Build history of the part. All positions in model axes, mm. A direction names the side the tool comes from. Round coordinates to 2 decimals unless told otherwise and drop trailing zeros. Order: outer loops, then holes, each group sorted by start corner. A loop starts at its lowest first (then second) coordinate and runs counter-clockwise, first axis right, second up. Notation, with made-up numbers: (-38.75, -3) -> (-14.75, -3) arc R18 cw to (-14.75, 11) -> close; hole circle Ø5 at (42.5, 11). An arc over 180 degrees is marked (long way). Use a Markdown table: item, result. Add a question column.
Item 1: Probe L1, parallel to X at y = 13.5, z = -88; L2, parallel to Z at x = 91, y = 7; L3, parallel to X at y = 25, z = -105. List the from-to ranges inside material, lowest first.
Item 2: Two-plate mould, pull along X, no slides. Class faces 6 (the face through (1, 4, -74)), 7 (the face through (74, 35, -54)): released by +X, released by -X, zero draft, split by the parting line, or undercut.
Item 3: Slice it at B-B, the plane z = -33. Give the cut face in (x, y).
Item 4: Pin check, flat tips, straight feed: pin 1 (2.5 mm diameter, centred on x = 1, y = 4.5, fed in from +Z); pin 2 (2 mm diameter, centred on y = 11, z = -59.5, fed in from -X); pin 3 (16 mm diameter, centred on x = 12, y = 8.5, fed in from +Z); pin 4 (1.2 mm diameter, centred on x = 29.5, z = -104.5, fed in from -Y). Stop position of each tip, or through.
Item 5: Slice it at A-A, the plane x = 62.5. Give the cut face in (y, z), plus the area to 3 significant figures.
Item 6: Slice it at D-D, the plane z = -53. Give the cut face in (x, y), plus the area to 3 significant figures.
Item 7: 3-axis set-ups, long thin cutter, end or side, ignore diameter. For faces 1 (the face through (5, 16, -106)), 2 (the face through (125, 16, -9)), 3 (the face through (1.52, 21.88, -86.65)), 4 (the face through (125, 35, -5)), 5 (the face through (59, 20.62, -1)): which of +Z, -Z, +X, -X, +Y, -Y reach the whole face in a straight line?
Item 8: Slice it at C-C, the plane x = 102.5. Give the cut face in (y, z), plus the area to 3 significant figures.
from build123d import *

# Parameters (mm, degrees)
SKETCH1_W           = 150
SKETCH1_H           = 110
BOSS_EXTRUDE1_DEPTH = 38
SKETCH3_W           = 144
SKETCH3_H           = 104
CUT_EXTRUDE1_DEPTH  = 35
CUT_EXTRUDE2_REACH  = 191.853
SKETCH5_W           = 10.5
SKETCH5_H           = 8.5
FILLET4_R           = 3
CUT_EXTRUDE3_REACH  = 191.853
SKETCH6_W           = 34.1
SKETCH6_H           = 45.2
CUT_EXTRUDE4_REACH  = 191.853
SKETCH10_W          = 15.12
SKETCH10_H          = 13.75
FILLET5_R           = 2
BOSS_EXTRUDE2_REACH = 191.853
SKETCH12_W          = 9
SKETCH12_H          = 6
SKETCH13_R          = 2.032
CUT_EXTRUDE5_DEPTH  = 35
CUT_EXTRUDE6_REACH  = 191.853
SKETCH14_W          = 28.8
SKETCH14_H          = 11
FILLET6_R           = 5
FILLET7_R           = 2
FILLET8_DEPTH       = 35
FILLET8_2_DEPTH     = 36
FILLET9_R           = 3


with BuildPart() as part:
    # Sketch1 → Boss-Extrude1 (new body)
    with BuildSketch(Plane(origin=(0, 0, 0), x_dir=(1, 0, 0), z_dir=(0, 1, 0))):
        with Locations((75, 55)):
            Rectangle(SKETCH1_W, SKETCH1_H)
    extrude(amount=BOSS_EXTRUDE1_DEPTH)

    # Sketch3 → Cut-Extrude1 (cut)
    with BuildSketch(Plane.XZ):
        with Locations((75, -55)):
            Rectangle(SKETCH3_W, SKETCH3_H)
    extrude(amount=-CUT_EXTRUDE1_DEPTH, mode=Mode.SUBTRACT)

    # Sketch5 → Cut-Extrude2 (cut, up to next)
    with BuildSketch(Plane.ZY, mode=Mode.PRIVATE) as cut_extrude2_sk1:
        with Locations((-91, 25.27)):
            Rectangle(SKETCH5_W, SKETCH5_H)
    cut_extrude2_tool1 = extrude(cut_extrude2_sk1.sketch, amount=-CUT_EXTRUDE2_REACH, mode=Mode.PRIVATE) & part.part
    add(cut_extrude2_tool1.solids().sort_by_distance((0, 25.27, -91))[0], mode=Mode.SUBTRACT)

    # Fillet4
    fillet4_edges = [part.edges().sort_by_distance(p)[0] for p in [
        (1.5, 21.02, -85.75),
        (1.5, 29.52, -85.75),
        (1.5, 29.52, -96.25),
        (1.5, 21.02, -96.25),
    ]]
    fillet(fillet4_edges, radius=FILLET4_R)

    # Sketch6 → Cut-Extrude3 (cut, up to next)
    with BuildSketch(Plane(origin=(0, 38, 0), x_dir=(1, 0, 0), z_dir=(0, 1, 0)), mode=Mode.PRIVATE) as cut_extrude3_sk1:
        with Locations((17.05, 22.6)):
            Rectangle(SKETCH6_W, SKETCH6_H)
    cut_extrude3_tool1 = extrude(cut_extrude3_sk1.sketch, amount=-CUT_EXTRUDE3_REACH, mode=Mode.PRIVATE) & part.part
    add(cut_extrude3_tool1.solids().sort_by_distance((17.05, 38, -22.6))[0], mode=Mode.SUBTRACT)

    # Sketch10 → Cut-Extrude4 (cut, up to next)
    with BuildSketch(Plane.XY, mode=Mode.PRIVATE) as cut_extrude4_sk1:
        with Locations((59.48, 13.745)):
            Rectangle(SKETCH10_W, SKETCH10_H)
    cut_extrude4_tool1 = extrude(cut_extrude4_sk1.sketch, amount=-CUT_EXTRUDE4_REACH, mode=Mode.PRIVATE) & part.part
    add(cut_extrude4_tool1.solids().sort_by_distance((59.48, 13.745, 0))[0], mode=Mode.SUBTRACT)

    # Fillet5
    fillet5_edges = [part.edges().sort_by_distance(p)[0] for p in [
        (51.92, 6.87, -1.5),
        (51.92, 20.62, -1.5),
        (67.04, 20.62, -1.5),
        (67.04, 6.87, -1.5),
    ]]
    fillet(fillet5_edges, radius=FILLET5_R)

    # Sketch12 → Boss-Extrude2 (add, up to next)
    with BuildSketch(Plane.XZ, mode=Mode.PRIVATE) as boss_extrude2_sk1:
        with Locations((125, -6)):
            Rectangle(SKETCH12_W, SKETCH12_H)
    boss_extrude2_tool1 = extrude(boss_extrude2_sk1.sketch, amount=-BOSS_EXTRUDE2_REACH, mode=Mode.PRIVATE) - part.part
    # Sketch12 → Boss-Extrude2 (add, up to next)
    with BuildSketch(Plane.XZ, mode=Mode.PRIVATE) as boss_extrude2_sk2:
        with Locations((30, -104)):
            Rectangle(SKETCH12_W, SKETCH12_H)
    boss_extrude2_tool2 = extrude(boss_extrude2_sk2.sketch, amount=-BOSS_EXTRUDE2_REACH, mode=Mode.PRIVATE) - part.part
    # Sketch12 → Boss-Extrude2 (add, up to next)
    with BuildSketch(Plane.XZ, mode=Mode.PRIVATE) as boss_extrude2_sk3:
        with Locations((125, -104)):
            Rectangle(SKETCH12_W, SKETCH12_H)
    boss_extrude2_tool3 = extrude(boss_extrude2_sk3.sketch, amount=-BOSS_EXTRUDE2_REACH, mode=Mode.PRIVATE) - part.part
    add(boss_extrude2_tool1.solids().sort_by_distance((125, 0, -6))[0])
    add(boss_extrude2_tool2.solids().sort_by_distance((30, 0, -104))[0])
    add(boss_extrude2_tool3.solids().sort_by_distance((125, 0, -104))[0])

    # Sketch13 → Cut-Extrude5 (cut)
    with BuildSketch(Plane.XZ):
        with Locations(Location((125, -5, 0), (0, 0, 270))):
            Circle(SKETCH13_R)
        with Locations(Location((125, -105, 0), (0, 0, 270))):
            Circle(SKETCH13_R)
        with Locations(Location((30, -105, 0), (0, 0, 270))):
            Circle(SKETCH13_R)
    extrude(amount=-CUT_EXTRUDE5_DEPTH, mode=Mode.SUBTRACT)

    # Sketch14 → Cut-Extrude6 (cut, up to next)
    with BuildSketch(Plane.ZY, mode=Mode.PRIVATE) as cut_extrude6_sk1:
        with Locations((-59.6, 5.5)):
            Rectangle(SKETCH14_W, SKETCH14_H)
    cut_extrude6_tool1 = extrude(cut_extrude6_sk1.sketch, amount=-CUT_EXTRUDE6_REACH, mode=Mode.PRIVATE) & part.part
    add(cut_extrude6_tool1.solids().sort_by_distance((0, 5.5, -59.6))[0], mode=Mode.SUBTRACT)

    # Fillet6
    fillet6_edges = [part.edges().sort_by_distance(p)[0] for p in [
        (147, 17.5, -3),
        (147, 17.5, -107),
        (3, 17.5, -107),
        (34.1, 36.5, -45.2),
        (0, 19, -110),
        (150, 19, -110),
        (150, 19, 0),
    ]]
    fillet(fillet6_edges, radius=FILLET6_R)

    # Fillet7
    fillet7_edges = [part.edges().sort_by_distance(p)[0] for p in [
        (1.5, 11, -74),
        (1.5, 11, -45.2),
    ]]
    fillet(fillet7_edges, radius=FILLET7_R)

    # Fillet8: read off the stored shape, not the designer's step
    # Fillet8 outline → Fillet8 (cut)
    with BuildSketch(Plane(origin=(0, 0, 0), x_dir=(1, 0, 0), z_dir=(0, 1, 0))):
        with BuildLine():
            Line((129.5, 101), (129.5, 104))
            ThreePointArc((129.5, 104), (128.621320344, 101.878679656), (126.5, 101))
            Line((126.5, 101), (129.5, 101))
        make_face()
        with BuildLine():
            Line((25.5, 101), (28.5, 101))
            ThreePointArc((28.5, 101), (26.378679656, 101.878679656), (25.5, 104))
            Line((25.5, 104), (25.5, 101))
        make_face()
        with BuildLine():
            Line((34.5, 101), (34.5, 104))
            ThreePointArc((34.5, 104), (33.621320344, 101.878679656), (31.5, 101))
            Line((31.5, 101), (34.5, 101))
        make_face()
        with BuildLine():
            Line((120.5, 101), (123.5, 101))
            ThreePointArc((123.5, 101), (121.378679656, 101.878679656), (120.5, 104))
            Line((120.5, 104), (120.5, 101))
        make_face()
        with BuildLine():
            Line((120.5, 9), (120.5, 6))
            ThreePointArc((120.5, 6), (121.378679656, 8.121320344), (123.5, 9))
            Line((123.5, 9), (120.5, 9))
        make_face()
        with BuildLine():
            Line((129.5, 9), (126.5, 9))
            ThreePointArc((126.5, 9), (128.621320344, 8.121320344), (129.5, 6))
            Line((129.5, 6), (129.5, 9))
        make_face()
    extrude(amount=FILLET8_DEPTH, mode=Mode.SUBTRACT)

    # Fillet8 2 outline → Fillet8 2 (add)
    with BuildSketch(Plane(origin=(0, 0, 0), x_dir=(1, 0, 0), z_dir=(0, 1, 0))):
        with BuildLine():
            Line((129.5, 107), (129.5, 104))
            ThreePointArc((129.5, 104), (130.378679656, 106.121320344), (132.5, 107))
            Line((132.5, 107), (129.5, 107))
        make_face()
        with BuildLine():
            ThreePointArc((22.5, 107), (24.621320344, 106.121320344), (25.5, 104))
            Line((25.5, 104), (25.5, 107))
            Line((25.5, 107), (22.5, 107))
        make_face()
        with BuildLine():
            ThreePointArc((34.5, 104), (35.378679656, 106.121320344), (37.5, 107))
            Line((37.5, 107), (34.5, 107))
            Line((34.5, 107), (34.5, 104))
        make_face()
        with BuildLine():
            ThreePointArc((117.5, 107), (119.621320344, 106.121320344), (120.5, 104))
            Line((120.5, 104), (120.5, 107))
            Line((120.5, 107), (117.5, 107))
        make_face()
        with BuildLine():
            Line((120.5, 3), (120.5, 6))
            ThreePointArc((120.5, 6), (119.621320344, 3.878679656), (117.5, 3))
            Line((117.5, 3), (120.5, 3))
        make_face()
        with BuildLine():
            ThreePointArc((132.5, 3), (130.378679656, 3.878679656), (129.5, 6))
            Line((129.5, 6), (129.5, 3))
            Line((129.5, 3), (132.5, 3))
        make_face()
    extrude(amount=FILLET8_2_DEPTH)

    # Fillet9
    fillet9_edges = [part.edges().sort_by_distance(p)[0] for p in [
        (147, 35, -55),
        (137.25, 35, -3),
        (15.25, 35, -107),
        (4.464466094, 35, -105.535533906),
        (145.535533906, 35, -4.464466094),
        (145.535533906, 35, -105.535533906),
        (125, 35, -101),
        (77.5, 35, -107),
        (137.25, 35, -107),
        (125, 35, -9),
        (75.8, 35, -3),
        (30, 35, -101),
        (24.621320344, 35, -106.121320344),
        (130.378679656, 35, -106.121320344),
        (130.378679656, 35, -3.878679656),
        (119.621320344, 35, -3.878679656),
        (35.378679656, 35, -106.121320344),
        (119.621320344, 35, -106.121320344),
        (128.621320344, 35, -101.878679656),
        (121.378679656, 35, -101.878679656),
        (33.621320344, 35, -101.878679656),
        (121.378679656, 35, -8.121320344),
        (128.621320344, 35, -8.121320344),
        (26.378679656, 35, -101.878679656),
        (3, 35, -73.6),
    ]]
    fillet(fillet9_edges, radius=FILLET9_R)


solid = part.part
Check sheet entries:
| question | item | result |
|---|---|---|
| 1 | L1 | 0 to 3, 147 to 150 |
| 1 | L2 | -110 to -107, -3 to 0 |
| 1 | L3 | 0 to 4, 25.33 to 27.97, 32.03 to 34.67, 120.33 to 122.97, 127.03 to 129.67, 146 to 150 |
| 2 | face 6 | zero draft |
| 2 | face 7 | undercut |
| 3 | outline | (34.1, 35) -> (144, 35) arc R3 cw to (147, 32) -> (147, 0) -> (150, 0) -> (150, 38) -> (34.1, 38) -> close |
| 4 | pin 1 | z = -74 |
| 4 | pin 2 | x = 0 |
| 4 | pin 3 | z = -105 |
| 4 | pin 4 | y = 35 |
| 5 | outline | (0, -110) -> (38, -110) -> (38, 0) -> (20.62, 0) -> (20.62, -3) -> (32, -3) arc R3 cw to (35, -6) -> (35, -104) arc R3 cw to (32, -107) -> (0, -107) -> close; (0, -3) -> (6.87, -3) -> (6.87, 0) -> (0, 0) -> close |
| 5 | area | 503 mm2 |
| 6 | outline | (0, 11) -> (3, 11) -> (3, 32) arc R3 cw to (6, 35) -> (144, 35) arc R3 cw to (147, 32) -> (147, 0) -> (150, 0) -> (150, 38) -> (0, 38) -> close |
| 6 | area | 631 mm2 |
| 7 | face 1 | +Z, -Y |
| 7 | face 2 | -X, -Y |
| 7 | face 3 | -X |
| 7 | face 4 | -Y |
| 7 | face 5 | +Z |
| 8 | outline | (0, -110) -> (38, -110) -> (38, 0) -> (0, 0) -> (0, -3) -> (32, -3) arc R3 cw to (35, -6) -> (35, -104) arc R3 cw to (32, -107) -> (0, -107) -> close |
| 8 | area | 544 mm2 |
